from build123d import *

# Parameters (mm, degrees)
SKETCH1_W               = 96
SKETCH1_H               = 75
BOSS_EXTRUDE1_DEPTH     = 65
SKETCH2_W               = 67
SKETCH2_H               = 104.92040837
CUT_EXTRUDE1_DEPTH      = 90.080020207
CUT_EXTRUDE2_DEPTH      = 111.785829419
CUT_EXTRUDE2_DEPTH_BACK = 111.785829419
SKETCH3_R               = 12.75
FILLET1_R               = 10


with BuildPart() as part:
    # Sketch1 → Boss-Extrude1 (new body)
    with BuildSketch(Plane.XY):
        Rectangle(SKETCH1_W, SKETCH1_H)
    extrude(amount=BOSS_EXTRUDE1_DEPTH)

    # Sketch2 → Cut-Extrude1 (cut, through all)
    with BuildSketch(Plane.XY.offset(65)):
        with Locations((0, 37.5)):
            Rectangle(SKETCH2_W, SKETCH2_H)
    extrude(amount=-CUT_EXTRUDE1_DEPTH, mode=Mode.SUBTRACT)

    # Sketch3 → Cut-Extrude2 (cut, two sides: drawn at the far end of the back side and taken through both)
    with BuildSketch(Plane(origin=(-33.5, 0, 0), x_dir=(0, 0, -1), z_dir=(1, 0, 0)).offset(-CUT_EXTRUDE2_DEPTH_BACK)):
        with Locations((-32.5, 17.878893252)):
            Circle(SKETCH3_R)
    extrude(amount=CUT_EXTRUDE2_DEPTH + CUT_EXTRUDE2_DEPTH_BACK, mode=Mode.SUBTRACT)

    # Fillet1
    fillet1_edges = [part.edges().sort_by_distance(p)[0] for p in [
        (-40.75, 37.5, 0),
        (-40.75, 37.5, 65),
        (-33.5, -14.960204185, 32.5),
        (33.5, -14.960204185, 32.5),
        (40.75, 37.5, 0),
        (40.75, 37.5, 65),
    ]]
    fillet(fillet1_edges, radius=FILLET1_R)


solid = part.part
The listing builds one solid part. Answer for the finished solid, in the listing's coordinates (mm). A direction names the side the tool comes from. Round coordinates to 2 decimals unless told otherwise and drop trailing zeros. Write each loop counter-clockwise with the first axis right and the second up, starting at its lowest first coordinate (ties: lowest second). Pieces come first, ordered by that corner, then holes. Notation, with made-up numbers: M 82.5,33 L 87.5,33 A19 cw 87.5,42 Z; hole C 23.25,-8 d5. An arc over 180 degrees is marked long. Write each question's results on one line, items separated by ' | '. Start each with the question number.
Item 1: Find section A-A on z = 32.5. Write down the section's boundary in (x, y).
Item 2: Find section B-B on y = -1. Write down the section's boundary in (x, z), and give its area (4 significant figures).
Item 3: Given pin 1 Ø6 at (x, z) = (-13, 16.5) entering from +Y, flat-ended and moving along its own axis, determine where the tip first touches the part or whether it passes through.
Item 4: Find section C-C on y = 9. Write down the section's boundary in (x, z), and give its area (3 significant figures).
Item 5: Find section D-D on x = 36. Write down the section's boundary in (y, z), and give its area (3 significant figures).
Item 6: Which of the six approach directions +Z, -Z, +X, -X, +Y, -Y give full straight-line access (tool end or side, diameter ignored) to faces 1 (the flat face through (-48, -1, 32)), 2 (the flat face through (-33.5, 6.5, 25.7))?
Item 7: Straight lines are drawn through the part: probe 1 along X at (y, z) = (10, 17); probe 2 along Y at (x, z) = (43.25, 32.5); probe 3 along Y at (x, z) = (-19.5, 58). For each, find the intervals that lie inside material, in ascending order.
Item 8: The mould has two halves that part along Z. Classify faces 3 (the cylindrical face through (-40.9, 10.1, 42.6)), 4 (the cylindrical face through (-30.6, -12, 32)), 5 (the cylindrical face through (-40.65, 34.49, 62.15)): +Z half, -Z half, draft (parallel to the pull), parting line (faces both ways), or undercut.
Answer block:
1) outline: M -48,-37.5 L 48,-37.5 L 48,5.13 L 33.5,5.13 L 33.5,-4.96 A10 cw 23.5,-14.96 L -23.5,-14.96 A10 cw -33.5,-4.96 L -33.5,5.13 L -48,5.13 Z; M -48,30.63 L -33.5,30.63 L -33.5,37.5 L -48,37.5 Z; M 33.5,30.63 L 48,30.63 L 48,37.5 L 33.5,37.5 Z
2) outline: M -48,0 L -33.5,0 L -33.5,65 L -48,65 Z; M 33.5,0 L 48,0 L 48,65 L 33.5,65 Z | area: 1,885 mm²
3) pin 1: stops at y = -14.96
4) outline: M -48,0 L -33.5,0 L -33.5,23.35 L -48,23.35 Z; M -48,41.65 L -33.5,41.65 L -33.5,65 L -48,65 Z; M 33.5,0 L 48,0 L 48,23.35 L 33.5,23.35 Z; M 33.5,41.65 L 48,41.65 L 48,65 L 33.5,65 Z | area: 1,350 mm²
5) outline: M -37.5,0 L 27.5,0 A10 ccw 37.5,10 L 37.5,55 A10 ccw 27.5,65 L -37.5,65 Z; hole C 17.88,32.5 d25.5 | area: 4,320 mm²
6) face 1: +Z, -Z, -X, +Y, -Y | face 2: +Z, -Z, +Y
7) probe 1: x = -48 to -33.5, 33.5 to 48 | probe 2: y = -37.5 to 5.13, 30.63 to 37.5 | probe 3: y = -37.5 to -14.96
8) face 3: undercut | face 4: draft | face 5: +Z half
